Autodesk Inventor part; units mm, degrees
ref_plane "Work Plane1" through (0, 120, 0) normal (0, 1, 0) x (-1, 0, 0)
ref_plane "Work Plane2" through (0, 0, 195) normal (0, 0, 1) x (1, 0, 0)
ref_plane "YZ Plane" through (0, 0, 0) normal (1, 0, 0) x (0, 1, 0)
sketch "Sketch1" plane through (0, 0, 0) normal (0, 0, 1) x (1, 0, 0)
  circle A0 centre (0, 0) radius 50
  dimension "d0" = 100
extrude "Extrusion1" add sketch "Sketch1" along normal blind 205
sketch "Sketch2" plane through (0, 0, 0) normal (1, 0, 0) x (0, 1, 0)
  line L0 (-50, 0) -> (50, 0) construction
  line L1 (0, 0) -> (0, -80)
  line L2 (0, -80) -> (35, -80)
  line L3 (0, 0) -> (5, 0)
  line L4 (5, 0) -> (5, -3.5)
  line L5 (9, -7.5) -> (45, -7.5)
  line L6 (45, -7.5) -> (45, -12.5)
  line L7 (45, -12.5) -> (35, -80)
  arc A0 (5, -3.5) -> (9, -7.5) centre (9, -3.5) ccw
  point P0 (5, -7.5)
  dimension "d3" = 80
  dimension "d4" = 35
  dimension "d5" = 5
  dimension "d6" = 7.5
  dimension "d7" = 40
  dimension "d8" = 5
  dimension "d9" = 4
revolve "Revolution1" add sketch "Sketch2" angle 360 about axis through (0, 0, 0) along (0, 0, -1)
ref_plane "Work Plane1" through (0, 120, 0) normal (0, 1, 0) x (-1, 0, 0)
sketch "Sketch3" plane through (0, 120, 0) normal (0, 1, 0) x (-1, 0, 0)
  line L0 (-50, 0) -> (50, 0) construction
  circle A0 centre (0, 45) radius 40
  line L1 (-50, 0) -> (-50, 205) construction
  point P0 (0, 0)
  dimension "d19" = 80
  dimension "d20" = 45
  dimension "d21" = 50
extrude "Extrusion2" add sketch "Sketch3" against normal blind 90
ref_plane "Work Plane2" through (0, 0, 195) normal (0, 0, 1) x (1, 0, 0)
sketch "Sketch4" plane through (0, 0, 195) normal (0, 0, 1) x (1, 0, 0)
  circle A0 centre (0, -60) radius 50 construction
  circle A1 centre (0, 0) radius 45 construction
  arc A2 (-44.9972, -0.4998) -> (44.9999, 0.1033) centre (0.0033, -0.4998) ccw
  line L0 (-50, -60) -> (50, -60)
  circle A3 centre (0, 0) radius 50 construction
  line L1 (-50, -60) -> (-50, 0)
  circle A4 centre (0, 0) radius 50 construction
  line L2 (50, -60) -> (50, 0)
  arc A5 (-50, 0) -> (50, 0) centre (0, 0) ccw
  point P0 (-44.9972, -38.1998)
  point P1 (44.9999, -81.7947)
  dimension "d26" = 100
  dimension "d27" = 60
  dimension "d29" = 90
extrude "Extrusion3" add sketch "Sketch4" against normal blind 5
sketch "Sketch7" plane through (0, 0, 0) normal (0, 0, -1) x (-1, 0, 0)
  line L0 (-50, -60) -> (50, -60) construction
  line L1 (50, -60) -> (50, 0) construction
  arc A0 (-50, 0) -> (50, 0) centre (0, 0) ccw construction
  line L2 (-50, 0) -> (-50, -60) construction
  line L3 (-50, -60) -> (50, -60)
  line L4 (50, -60) -> (50, 0)
  circle A1 centre (0, 0) radius 50 construction
  line L5 (-50, -60) -> (50, -60)
  line L6 (-50, 0) -> (-50, -60)
  line L7 (-50, -60) -> (-50, 0)
  arc A2 (-50, 0) -> (50, 0) centre (0, 0) ccw
extrude "Extrusion5" add sketch "Sketch7" against normal blind 5
sketch "Sketch8" plane through (0, 0, 0) normal (0, 0, -1) x (-1, 0, 0)
  line L0 (50, -60) -> (-50, -60)
  line L1 (50, 0) -> (50, -60) construction
  line L2 (-50, -60) -> (50, -60)
  line L3 (50, -60) -> (50, -57.5)
  line L4 (50, -57.5) -> (-50, -57.5)
  line L5 (-50, -57.5) -> (-50, -60)
  point P0 (0, 0)
  dimension "d37" = 2.5
extrude "Extrusion6" add sketch "Sketch8" along normal blind 20
sketch "Sketch9" plane through (-50, -57.5, 0) normal (0, 1, 0) x (1, 0, 0)
  circle A0 centre (20, 12.5) radius 5 construction
  circle A1 centre (80, 12.5) radius 5 construction
  line L0 (0, 0) -> (0, 20) construction
  line L1 (100, 0) -> (0, 0) construction
  point P0 (50, 0)
  dimension "d40" = 10
  dimension "d41" = 10
  dimension "d42" = 60
  dimension "d43" = 20
  dimension "d45" = 12.5
hole "Hole1" at (-30, -57.5, -12.5) at (30, -57.5, -12.5) direction (0, -1, 0) diameter 5 end through all
sketch "Sketch10" plane through (0, 0, 195) normal (0, 0, 1) x (1, 0, 0)
  line L0 (50, 0) -> (50, -60) construction
  line L1 (-50, -60) -> (50, -60)
  line L2 (50, -60) -> (50, -57.5)
  line L3 (50, -57.5) -> (-50, -57.5)
  line L4 (-50, -57.5) -> (-50, -60)
  point P0 (0, 0)
  dimension "d53" = 2.5
extrude "Extrusion7" add sketch "Sketch10" along normal blind 25
sketch "Sketch11" plane through (-50, -57.5, 195) normal (0, 1, 0) x (1, 0, 0)
  circle A0 centre (20, -17.5) radius 5 construction
  circle A1 centre (80, -17.5) radius 5 construction
  line L0 (100, -25) -> (0, -25) construction
  line L1 (0, 0) -> (0, -25) construction
  point P0 (50, 195)
  dimension "d56" = 10
  dimension "d57" = 10
  dimension "d58" = 7.5
  dimension "d59" = 20
  dimension "d60" = 60
hole "Hole2" at (-30, -57.5, 212.5) at (30, -57.5, 212.5) direction (0, -1, 0) diameter 5 end through all
fillet "Fillet1" radius 2 9 edges at (-50, 0, 205) (-50, -58.75, 220) (50, -58.75, 220) (-50, -58.75, -20) (50, -58.75, -20) (0, -60, 5) (0, -60, 190) (0, -35, -80) (40, 120, 45)
properties part number "Compressor_PX06" material "Polyethylene, High Density"
Source: CAD feature listing. Evaluate the final solid. Frame: model axes, mm. A direction names the side the tool comes from. Give positions to 0.01 mm unless a question says otherwise; leave off trailing zeros. Write each loop counter-clockwise with the first axis right and the second up, starting at its lowest first coordinate (ties: lowest second). Pieces come first, ordered by that corner, then holes. Notation, with made-up numbers: (-15.5, 59.5) -> (7.5, 59.5) arc R36 cw to (7.5, 98.5) -> close; hole circle Ø5 at (72.25, 70). An arc over 180 degrees is marked (long way). Return JSON: item names as keys, results as strings. Group by question number.
1. Access query for faces 1 (the face through (-39.923, 20.765, -10.035)), 2 (the face through (-0.2, -50.3, 190)), 3 (the face through (1, -57.5, 207)). Directions: +Z, -Z, +X, -X, +Y, -Y. A direction counts if a zero-diameter tool reaches every point of the face in a straight line with its end or side. Return the directions, or none.
2. Section A-A, the plane z = 45. Output: boundary loops of the cut face in (x, y).
3. Section B-B, the plane y = 98. Output: boundary loops of the cut face in (x, z).
4. Mould query, pull axis Y, two halves, no side actions, for faces 4 (the face through (-1, -60, 206)), 5 (the face through (-21.5, 74.61, 78.73)), 6 (the face through (-1, -57.5, -10)), 7 (the face through (1, 120, 46)). Classes: +Y half, -Y half, draft (parallel to the pull), parting line (faces both ways), or undercut.
5. Pin query (flat end, axial travel): pin 1 Ø20 at (x, z) = (3.5, 203.5) entering from +Y; pin 2 Ø10 at (x, z) = (3, -10.5) entering from +Y; pin 3 Ø2 at (x, z) = (1, 132) entering from -Y. Return the tip coordinate at first contact, or that it passes through.
6. Section C-C, the plane z = 131.5. Output: boundary loops of the cut face in (x, y).
7. Material intervals for line 1 (X direction, y = -58.55, z = -12.5); line 2 (Z direction, x = 30, y = -58); line 3 (Z direction, x = 22, y = 17.5), sorted ascending. Write a range as from..to.
Determined:
{
 "1": {"face 1": "-Z", "face 2": "-Y", "face 3": "+Z, +X, -X"},
 "2": {"outline": "(-40, 30) arc R50 ccw (long way) to (40, 30) -> (40, 118) arc R2 ccw to (38, 120) -> (-38, 120) arc R2 ccw to (-40, 118) -> close"},
 "3": {"outline": "circle Ø80 at (0, 45)"},
 "4": {"face 4": "-Y half", "face 5": "draft", "face 6": "undercut", "face 7": "+Y half"},
 "5": {"pin 1": "stops at y = 50", "pin 2": "stops at y = 45", "pin 3": "stops at y = -50"},
 "6": {"outline": "circle Ø100 at (0, 0)"},
 "7": {"line 1": "x = -50..-32.5, -27.5..27.5, 32.5..50", "line 2": "z = -20..-15, -10..5, 190..210, 215..220", "line 3": "z = -80..-7.5, 0..205"}
}
